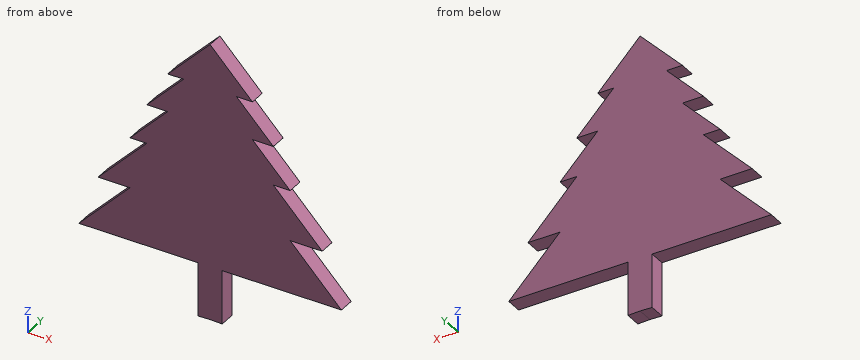
from build123d import *

# Parameters (mm, degrees)
F1_DEPTH = 6.35


with BuildPart() as f1:
    # F0 (on Front) → F1 (new body)
    with BuildSketch(Plane.XZ):
        Polygon((16.844211, 50.833423), (0, 68.279214), (-16.844211, 50.833423), (-10.527632, 50.833423), (-25.174322, 35.663635), (-16.844211, 35.663635), (-31.850775, 20.121122), (-25.174322, 20.121122), (-44.60161, 0), (-31.850775, 0), (-52.245557, -21.123168), (-4.812632, -21.123168), (-4.812632, -42.596416), (0, -42.411316), (4.812632, -42.596416), (4.812632, -21.123168), (52.245557, -21.123168), (31.850775, 0), (44.60161, 0), (25.174322, 20.121122), (31.850775, 20.121122), (16.844211, 35.663635), (25.174322, 35.663635), (10.527632, 50.833423), align=None)
    extrude(amount=F1_DEPTH)


solid = f1.part
Can you work these out from the model? Positions are in its coordinate system, mm. Coordinates: 2 decimals unless noted, no trailing zeros. Write each loop counter-clockwise with the first axis right and the second up, starting at its lowest first coordinate (ties: lowest second). Pieces come first, ordered by that corner, then holes. Notation, with made-up numbers: M 4,37.25 L 10,37.25 A28 cw 10,69.25 Z; hole C 46,-35 d6. An arc over 180 degrees is marked long. Use one line per item in the form item = value.
Q1. If we section it at D-D (x = 19): Write out the boundary of the cut face in (y, z), then the cut area to 3 significant figures.
Model answer:
outline = M -6.35,-21.12 L 0,-21.12 L 0,33.43 L -6.35,33.43 Z; M -6.35,35.66 L 0,35.66 L 0,42.06 L -6.35,42.06 Z
area = 387 mm^2
Q2. I need wall thicknesses on line 1 along Z through (x, y) = (-30.5, -5); line 2 along Z through (x, y) = (37, -5); line 3 along X through (y, z) = (-1.5, -36.5). Which ranges of each line are inside material? Lowest first, please. Write a range as from..to.
Model answer:
line_1 = -21.12..14.61, 20.12..21.52
line_2 = -21.12..-5.33, 0..7.87
line_3 = -4.81..4.81
Q3. If we section it at C-C (z = -29): Write out the boundary of the cut face in (x, y), then the cut area to 3 significant figures.
Model answer:
outline = M -4.81,-6.35 L 4.81,-6.35 L 4.81,0 L -4.81,0 Z
area = 61.1 mm^2
Q4. If we section it at A-A (x = 33.5): Write out the boundary of the cut face in (y, z).
Model answer:
outline = M -6.35,-21.12 L 0,-21.12 L 0,-1.71 L -6.35,-1.71 Z; M -6.35,0 L 0,0 L 0,11.5 L -6.35,11.5 Z
Q5. For P1, Ø2, axis at x = -26, y = -2, coming from the -Z side; P2, Ø3, axis at y = -1.5, z = 24.5, coming from the -X side; P3, Ø1.9, axis at y = -3.5, z = -27.5, coming from the -X side, each with a flat end and sliding along its axis, tell me the tip position at first contact or that it passes through.
Model answer:
P1 = -21.12
P2 = -29.07
P3 = -4.81
Q6. If we section it at B-B (y = -2.75): Write out the boundary of the cut face in (x, z).
Model answer:
outline = M -52.25,-21.12 L -4.81,-21.12 L -4.81,-42.6 L 0,-42.41 L 4.81,-42.6 L 4.81,-21.12 L 52.25,-21.12 L 31.85,0 L 44.6,0 L 25.17,20.12 L 31.85,20.12 L 16.84,35.66 L 25.17,35.66 L 10.53,50.83 L 16.84,50.83 L 0,68.28 L -16.84,50.83 L -10.53,50.83 L -25.17,35.66 L -16.84,35.66 L -31.85,20.12 L -25.17,20.12 L -44.6,0 L -31.85,0 Z
